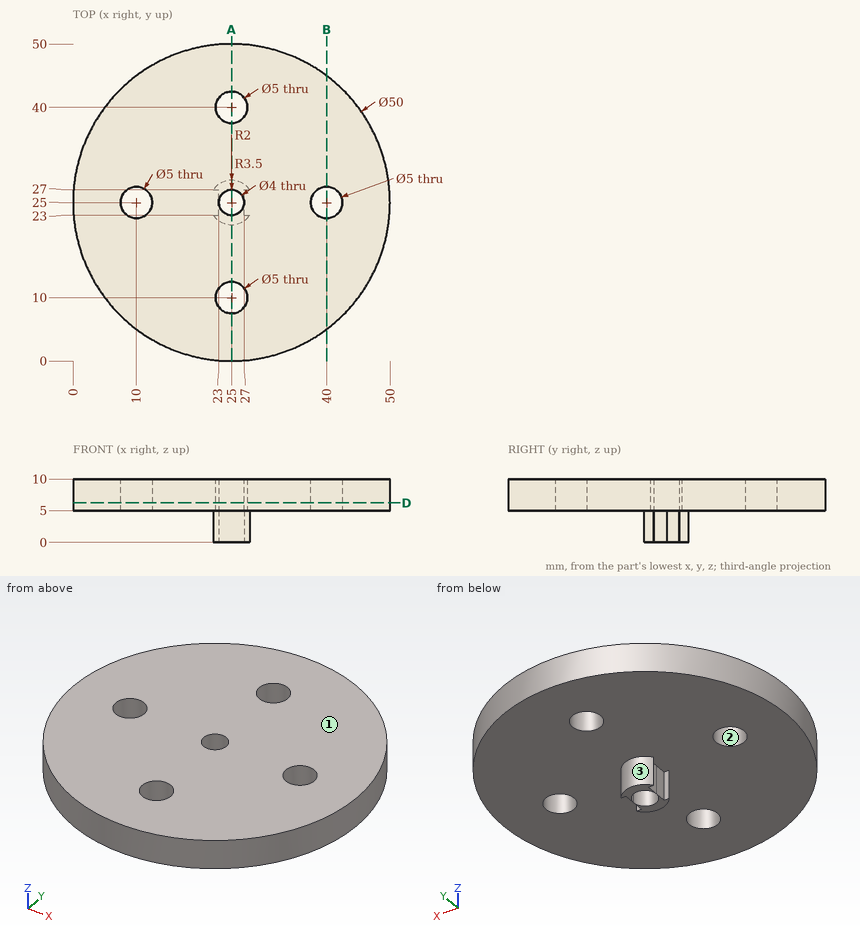
Here's the drawing with two shaded views (mm, measured from the low corner). I have some questions. Coordinates: 2 decimals unless noted, no trailing zeros. Write each loop counter-clockwise with the first axis right and the second up, starting at its lowest first coordinate (ties: lowest second). Pieces come first, ordered by that corner, then holes. Notation, with made-up numbers: (39, 45) - (51, 45) arc R33 cw to (51, 73) - close; hole circle Ø6 at (77, 52.25). An arc over 180 degrees is marked (long way). Return JSON: item names as keys, results as strings.
Q1. If we section it at A-A (x = 25): Please give me the cut outline in (y, z), then the cut area to 3 significant figures.
Computed values:
{"outline": "(0, 5) - (7.5, 5) - (7.5, 10) - (0, 10) - close; (12.5, 5) - (21.5, 5) - (21.5, 0) - (23, 0) - (23, 10) - (12.5, 10) - close; (27, 0) - (28.5, 0) - (28.5, 5) - (37.5, 5) - (37.5, 10) - (27, 10) - close; (42.5, 5) - (50, 5) - (50, 10) - (42.5, 10) - close", "area": "195 mm2"}
Q2. If we section it at B-B (x = 40): Please give me the cut outline in (y, z).
Computed values:
{"outline": "(5, 5) - (22.5, 5) - (22.5, 10) - (5, 10) - close; (27.5, 5) - (45, 5) - (45, 10) - (27.5, 10) - close"}
Q3. Thinking about a two-plate mould opening in X: for the marked faces 1, 2 and 3, which applies, +X half, -X half, draft (parallel to the pull), parting line (faces both ways), or undercut?
Computed values:
{"face 1": "draft", "face 2": "undercut", "face 3": "parting line"}
Q4. Please list where these lines run through material, in increasing order: L1, parallel to Y at x = 25, z = 8.2; L2, parallel to X at y = 24, z = 7.25; L3, parallel to Z at x = 18, y = 18. Write a range as from..to.
Computed values:
{"L1": "y = 0..7.5, 12.5..23, 27..37.5, 42.5..50", "L2": "x = 0.02..7.71, 12.29..23.27, 26.73..37.71, 42.29..49.98", "L3": "z = 5..10"}
Q5. I'm going to push flat-ended pins straight in: pin 1 Ø1 at (x, z) = (24.5, 5.5) entering from +Y; pin 2 Ø6 at (x, y) = (25, 40) entering from -Z; pin 3 Ø6 at (y, z) = (19.5, 6) entering from -X. Where does each tip first touch, or does it pass through?
Computed values:
{"pin 1": "stops at y = 50", "pin 2": "stops at z = 5", "pin 3": "stops at x = 0.13"}
Q6. If we section it at D-D (z = 6.25): Please give me the cut outline in (x, y).
Computed values:
{"outline": "circle Ø50 at (25, 25); hole circle Ø5 at (10, 25); hole circle Ø5 at (25, 10); hole circle Ø5 at (25, 40); hole circle Ø4 at (25, 25); hole circle Ø5 at (40, 25)"}
